Geometry check sheet. Reference: the model listing, model coordinates, mm. A direction names the side the tool comes from. Coordinates: 2 decimals unless noted, no trailing zeros. Order: outer loops, then holes, each group sorted by start corner. A loop starts at its lowest first (then second) coordinate and runs counter-clockwise, first axis right, second up. Notation, with made-up numbers: M 85,60.25 L 130,60.25 A23 cw 130,87.25 Z; hole C 41,22 d2. An arc over 180 degrees is marked long. Use CSV: the item, a comma, the result in double quotes. Start each with the question number.
```python
from build123d import *

# Parameters (mm, degrees)
SKETCH1_W           = 139.7
SKETCH1_H           = 25.4
BOSS_EXTRUDE1_DEPTH = 6.35
SKETCH2_R           = 6.35
BOSS_EXTRUDE2_DEPTH = 177.8
SKETCH3_R           = 1.27
CUT_EXTRUDE1_DEPTH  = 7.35


with BuildPart() as part:
    # Sketch1 → Boss-Extrude1 (new body)
    with BuildSketch(Plane(origin=(0, 0, 0), x_dir=(1, 0, 0), z_dir=(0, 1, 0))):
        with BuildLine():
            Line((-69.85, 12.7), (-69.85, -12.7))
            ThreePointArc((-69.85, -12.7), (-82.55, 0), (-69.85, 12.7))
        make_face()
        with BuildLine():
            ThreePointArc((69.85, 12.7), (82.55, 0), (69.85, -12.7))
            Line((69.85, -12.7), (69.85, 12.7))
        make_face()
        Rectangle(SKETCH1_W, SKETCH1_H)
    extrude(amount=BOSS_EXTRUDE1_DEPTH)

    # Sketch2 → Boss-Extrude2 (add)
    with BuildSketch(Plane(origin=(0, 6.35, 0), x_dir=(1, 0, 0), z_dir=(0, 1, 0))):
        with Locations((-69.85, 0)):
            Circle(SKETCH2_R)
        with Locations((69.85, 0)):
            Circle(SKETCH2_R)
    extrude(amount=BOSS_EXTRUDE2_DEPTH)

    # Sketch3 → Cut-Extrude1 (cut, through all)
    with BuildSketch(Plane(origin=(0, 6.35, 0), x_dir=(1, 0, 0), z_dir=(0, 1, 0))):
        with Locations((-10.16, 0)):
            Circle(SKETCH3_R)
        with Locations((10.16, 0)):
            Circle(SKETCH3_R)
    extrude(amount=-CUT_EXTRUDE1_DEPTH, mode=Mode.SUBTRACT)


solid = part.part
```
1) Gauge pin test, flat ends, axial feed: P1, Ø4, axis at x = -13, z = -6, coming from the +Y side; P2, Ø1, axis at y = 86.5, z = 0, coming from the +X side; P3, Ø3, axis at y = 161, z = 3, coming from the +X side. Record the tip position at first contact, or that the pin passes through.
2) Set-up check for faces 4 (the face through (75.907, 94.005, -1.907)), 5 (the face through (70, 184.15, 0)): record each of +Z, -Z, +X, -X, +Y, -Y from which the full face is reachable in a straight line by a thin tool's end or side.
3) Material ranges on line 1 along X through (y, z) = (5, 0); line 2 along Z through (x, y) = (-10.16, 2.5); line 3 along X through (y, z) = (48.5, 0), recorded low to high.
4) Section check C-C on x = 51.5. Record the boundary of the cut face in (y, z).
5) Section check A-A on y = 64. Record the boundary of the cut face in (x, z).
6) Draft check along X on faces 1 (the face through (1, 0, 0)), 2 (the face through (-82.547, 3.131, 0.279)), 3 (the face through (-63.984, 94.005, 2.432)). Enter one of: +X half, -X half, draft (parallel to the pull), parting line (faces both ways), or undercut.
7) Section check B-B on z = -4. Record the boundary of the cut face in (x, y).
Results are:
1,P1,"stops at y = 6.35"
1,P2,"stops at x = 76.2"
1,P3,"stops at x = 76.02"
2,face 4,"+Y"
2,face 5,"+Z, -Z, +X, -X, +Y"
3,line 1,"x = -82.55 to -11.43, -8.89 to 8.89, 11.43 to 82.55"
3,line 2,"z = -12.7 to -1.27, 1.27 to 12.7"
3,line 3,"x = -76.2 to -63.5, 63.5 to 76.2"
4,outline,"M 0,-12.7 L 6.35,-12.7 L 6.35,12.7 L 0,12.7 Z"
5,outline,"C -69.85,0 d12.7; C 69.85,0 d12.7"
6,face 1,"draft"
6,face 2,"-X half"
6,face 3,"undercut"
7,outline,"M -81.9,0 L 81.9,0 L 81.9,6.35 L 74.78,6.35 L 74.78,184.15 L 64.92,184.15 L 64.92,6.35 L -64.92,6.35 L -64.92,184.15 L -74.78,184.15 L -74.78,6.35 L -81.9,6.35 Z"
